```python
from build123d import *

# Parameters (mm, degrees)
SKETCH1_R           = 1.95
SKETCH1_R_2         = 4
SKETCH1_R_3         = 1.45
BOSS_EXTRUDE1_DEPTH = 3


with BuildPart() as part:
    # Sketch1 → Boss-Extrude1 (new body)
    with BuildSketch(Plane.XY.offset(-5.551615438)):
        with BuildLine():
            Line((-25.464626351, 10.13731735), (-12.396849296, 10.13731735))
            Line((-12.396849296, 10.13731735), (-12.396849296, 19.63731735))
            Line((-12.396849296, 19.63731735), (-7.414626351, 19.63731735))
            Line((-7.414626351, 19.63731735), (-7.414626351, 15.63731735))
            Line((-7.414626351, 15.63731735), (-8.864626351, 15.63731735))
            Line((-8.864626351, 15.63731735), (-8.864626351, 12.63731735))
            Line((-8.864626351, 12.63731735), (-7.414626351, 12.63731735))
            Line((-7.414626351, 12.63731735), (-7.414626351, 6.63731735))
            Line((-7.414626351, 6.63731735), (-3.514626351, 6.63731735))
            Line((-3.514626351, 6.63731735), (-3.514626351, 12.63731735))
            Line((-3.514626351, 12.63731735), (-2.064626351, 12.63731735))
            Line((-2.064626351, 12.63731735), (-2.064626351, 15.63731735))
            Line((-2.064626351, 15.63731735), (-3.514626351, 15.63731735))
            Line((-3.514626351, 15.63731735), (-3.514626351, 19.63731735))
            Line((-3.514626351, 19.63731735), (2.585373649, 19.63731735))
            Line((2.585373649, 19.63731735), (2.585373649, 15.63731735))
            Line((2.585373649, 15.63731735), (1.135373649, 15.63731735))
            Line((1.135373649, 15.63731735), (1.135373649, 12.63731735))
            Line((1.135373649, 12.63731735), (2.585373649, 12.63731735))
            Line((2.585373649, 12.63731735), (2.585373649, 6.63731735))
            Line((2.585373649, 6.63731735), (6.485373649, 6.63731735))
            Line((6.485373649, 6.63731735), (6.485373649, 12.63731735))
            Line((6.485373649, 12.63731735), (7.935373649, 12.63731735))
            Line((7.935373649, 12.63731735), (7.935373649, 15.63731735))
            Line((7.935373649, 15.63731735), (6.485373649, 15.63731735))
            Line((6.485373649, 15.63731735), (6.485373649, 19.63731735))
            Line((6.485373649, 19.63731735), (11.467596593, 19.63731735))
            Line((11.467596593, 19.63731735), (11.467596593, 10.13731735))
            Line((11.467596593, 10.13731735), (24.535373649, 10.13731735))
            ThreePointArc((24.535373649, 10.13731735), (25.949587211, 9.551530913), (26.535373649, 8.13731735))
            Line((26.535373649, 8.13731735), (26.535373649, -6.86268265))
            ThreePointArc((26.535373649, -6.86268265), (25.949587211, -8.276896212), (24.535373649, -8.86268265))
            Line((24.535373649, -8.86268265), (-10, -8.86268265))
            Line((-10, -8.86268265), (-25.464626351, -8.86268265))
            ThreePointArc((-25.464626351, -8.86268265), (-26.878839913, -8.276896212), (-27.464626351, -6.86268265))
            Line((-27.464626351, -6.86268265), (-27.464626351, 8.13731735))
            ThreePointArc((-27.464626351, 8.13731735), (-26.878839913, 9.551530913), (-25.464626351, 10.13731735))
        make_face()
        with Locations((-24.464626351, -4.36268265)):
            Circle(SKETCH1_R, mode=Mode.SUBTRACT)
        with Locations((23.535373649, -4.36268265)):
            Circle(SKETCH1_R, mode=Mode.SUBTRACT)
        with Locations((9.535373649, 0.63731735)):
            Circle(SKETCH1_R_2, mode=Mode.SUBTRACT)
        with Locations((-10.464626351, 0.63731735)):
            Circle(SKETCH1_R_3, mode=Mode.SUBTRACT)
        with Locations((-24.464626351, 2.63731735)):
            Circle(SKETCH1_R_3, mode=Mode.SUBTRACT)
        with Locations((23.535373649, 2.63731735)):
            Circle(SKETCH1_R_3, mode=Mode.SUBTRACT)
    extrude(amount=BOSS_EXTRUDE1_DEPTH)


solid = part.part
```
Geometry check sheet. Reference: the model listing, model coordinates, mm. A direction names the side the tool comes from. Coordinates: 2 decimals unless noted, no trailing zeros. Write each loop counter-clockwise with the first axis right and the second up, starting at its lowest first coordinate (ties: lowest second). Pieces come first, ordered by that corner, then holes. Notation, with made-up numbers: M 88.25,-14 L 114.25,-14 A33 ccw 114.25,22 Z; hole C 21.25,44.5 d6. An arc over 180 degrees is marked long. One line per item, written item: value. Start each with the question number.
(1) Sectioned sample at B-B, the plane x = -21. Enter the section's corners in (y, z).
(2) Sectioned sample at C-C, the plane y = 0. Enter the section's corners in (x, z).
(3) Sectioned sample at D-D, the plane z = -3.35. State how many separate pieces and enclosed holes the cut face has, and give its area (3 significant figures).
(4) Sectioned sample at A-A, the plane y = 16.25. Enter the section's corners in (x, z).
(5) Tool access check on faces 4 (the face through (-3, 15.637, -4)), 5 (the face through (-5, 6.637, -4)), 6 (the face through (25.9, 9.6, -4.1)). Record the directions out of +Z, -Z, +X, -X, +Y, -Y that give a thin tool (end or side, any length) a straight path to the whole face; none if there is none.
(6) Depth check by flat-ended pin: pin 1 (1.5 mm diameter, centred on y = 14.5, z = -4, fed in from +X); pin 2 (0.9 mm diameter, centred on x = 4, z = -4, fed in from +Y); pin 3 (2.5 mm diameter, centred on x = -24.46, y = 2.64, fed in from +Z); pin 4 (1.5 mm diameter, centred on y = 9.5, z = -3, fed in from -X). Enter the tip coordinate at first touch or a pass-through.
(7) Release check for a two-part mould opening along X. For faces 1 (the face through (2.585, 18, -4)), 2 (the face through (-27.465, 1, -4)), 3 (the face through (0, 2, -5.552)) record: released by +X, released by -X, zero draft, split by the parting line, or undercut.
(8) Scan lines: line 1 along X through (y, z) = (14.75, -4.9); line 2 along X through (y, z) = (18.25, -3.1); line 3 along Y through (x, z) = (23.5, -2.8). Record each from-to range of solid material in increasing order. Write a range as [from, to].
Filled sheet:
1. outline: M -8.86,-5.55 L 10.14,-5.55 L 10.14,-2.55 L -8.86,-2.55 Z
2. outline: M -27.46,-5.55 L -11.77,-5.55 L -11.77,-2.55 L -27.46,-2.55 Z; M -9.16,-5.55 L 5.59,-5.55 L 5.59,-2.55 L -9.16,-2.55 Z; M 13.48,-5.55 L 26.54,-5.55 L 26.54,-2.55 L 13.48,-2.55 Z
3. separate pieces: 1
3. enclosed holes: 6
3. area: 1,040 mm²
4. outline: M -12.4,-5.55 L -7.41,-5.55 L -7.41,-2.55 L -12.4,-2.55 Z; M -3.51,-5.55 L 2.59,-5.55 L 2.59,-2.55 L -3.51,-2.55 Z; M 6.49,-5.55 L 11.47,-5.55 L 11.47,-2.55 L 6.49,-2.55 Z
5. face 4: +Z, -Z
5. face 5: +Z, -Z, +Y
5. face 6: +Z, -Z, +X, +Y
6. pin 1: x = 11.47
6. pin 2: y = 6.64
6. pin 3: through
6. pin 4: x = -27.37
7. face 1: undercut
7. face 2: released by -X
7. face 3: zero draft
8. line 1: [-12.4, -8.86], [-2.06, 1.14], [7.94, 11.47]
8. line 2: [-12.4, -7.41], [-3.51, 2.59], [6.49, 11.47]
8. line 3: [-8.86, -6.31], [-2.41, 1.19], [4.09, 10.14]
